from build123d import *

# Parameters (mm, degrees)
SKETCH_1_W          = 99.999995276
SKETCH_1_H          = 99.999995276
SKETCH_1_R          = 7
EXTRUDE_2_DEPTH     = 4
FILLET_2_R          = 7
EXTRUDE_3_DEPTH     = 116
FILLET_3_R          = 3
FILLET_4_R          = 1
CUT_EXTRUDE_1_DEPTH = 116
RIB_1_REACH         = 141.284
SKETCH_6_WALL_W     = 331.945026876
SKETCH_6_WALL_H     = 3


with BuildPart() as part:
    # 草图1 → 凸台-拉伸2 (new body)
    with BuildSketch(Plane(origin=(0, 0, 0), x_dir=(1, 0, 0), z_dir=(0, 1, 0))):
        Rectangle(SKETCH_1_W, SKETCH_1_H)
        with Locations(Location((-35, 35, 0), (0, 0, 270))):
            Circle(SKETCH_1_R, mode=Mode.SUBTRACT)
        with Locations(Location((35, 35, 0), (0, 0, 270))):
            Circle(SKETCH_1_R, mode=Mode.SUBTRACT)
        with Locations(Location((35, -35, 0), (0, 0, 270))):
            Circle(SKETCH_1_R, mode=Mode.SUBTRACT)
        with Locations(Location((-35, -35, 0), (0, 0, 270))):
            Circle(SKETCH_1_R, mode=Mode.SUBTRACT)
    extrude(amount=EXTRUDE_2_DEPTH)

    # 圆角2
    fillet_2_edges = [part.edges().sort_by_distance(p)[0] for p in [
        (-49.999997638, 2, -49.999997638),
        (49.999997638, 2, -49.999997638),
        (49.999997638, 2, 49.999997638),
        (-49.999997638, 2, 49.999997638),
    ]]
    fillet(fillet_2_edges, radius=FILLET_2_R)

    # 草图3 → 凸台-拉伸3 (add)
    with BuildSketch(Plane(origin=(0, 4, 0), x_dir=(1, 0, 0), z_dir=(0, 1, 0))):
        Polygon((-21, -24), (-21, -21), (21, -21), (21, 21), (-21, 21), (-21, 24), (24, 24), (24, -24), align=None)
    extrude(amount=EXTRUDE_3_DEPTH)

    # 圆角3
    fillet_3_edges = [part.edges().sort_by_distance(p)[0] for p in [
        (-21, 120, 22.5),
        (-21, 120, -22.5),
    ]]
    fillet(fillet_3_edges, radius=FILLET_3_R)

    # 圆角4
    fillet_4_edges = [part.edges().sort_by_distance(p)[0] for p in [
        (24, 62, 24),
        (24, 62, -24),
        (21, 62, -21),
        (21, 62, 21),
    ]]
    fillet(fillet_4_edges, radius=FILLET_4_R)

    # 草图4 → 切除-拉伸1 (cut)
    with BuildSketch(Plane(origin=(0, 0, -24), x_dir=(-1, 0, 0), z_dir=(0, 0, -1))):
        with BuildLine():
            Line((4.5, 93.761812865), (4.5, 71.261812865))
            ThreePointArc((4.5, 71.261812865), (0, 66.761812865), (-4.5, 71.261812865))
            Line((-4.5, 71.261812865), (-4.5, 93.761812865))
            ThreePointArc((-4.5, 93.761812865), (0, 98.261812865), (4.5, 93.761812865))
        make_face()
        with BuildLine():
            Line((4.5, 42.026719912), (4.5, 19.526719912))
            ThreePointArc((4.5, 19.526719912), (0, 15.026719912), (-4.5, 19.526719912))
            Line((-4.5, 19.526719912), (-4.5, 42.026719912))
            ThreePointArc((-4.5, 42.026719912), (0, 46.526719912), (4.5, 42.026719912))
        make_face()
    extrude(amount=-CUT_EXTRUDE_1_DEPTH, mode=Mode.SUBTRACT)

    # 草图6 wall → 筋1 (add, up to next)
    with BuildSketch(Plane(origin=(35.249998819, 27.094227832, 0), x_dir=(0.437936853183, -0.89900573559, 0), z_dir=(0.89900573559, 0.437936853183, 0)), mode=Mode.PRIVATE) as rib_1_sk1:
        Rectangle(SKETCH_6_WALL_W, SKETCH_6_WALL_H)
    rib_1_tool1 = extrude(rib_1_sk1.sketch, amount=-RIB_1_REACH, mode=Mode.PRIVATE) - part.part
    add(rib_1_tool1.solids().sort_by_distance((35.249998819, 27.094227832, 0))[0])


solid = part.part
Input: part model. Units: mm. Frame: model coordinates. A direction names the side the tool comes from. Coordinates: 2 decimals unless noted, no trailing zeros. Loops run counter-clockwise (first coordinate to the right, second up) from the corner with the lowest first, then second, coordinate; pieces in that order, holes last. Notation, with made-up numbers: (54, 12.5) -> (74, 12.5) arc R20 ccw to (74, 31.5) -> close; hole circle Ø6 at (30, 10). An arc over 180 degrees is marked (long way). Write item = value, one per line. Start each with the question number.
Item 1: Cut plane A-A, the plane x = 0. Return loops of the section in (y, z), plus the area to 3 significant figures.
Item 2: First-contact query: P1, Ø2.5, axis at y = 25, z = 22.5, coming from the +X side; P2, Ø0.9, axis at y = 26.5, z = -22, coming from the -X side; P3, Ø12, axis at x = 9.5, y = 36.5, coming from the +Z side; P4, Ø12.5, axis at x = 35, z = 35, coming from the +Y side. Flat tips, straight axial feed; report the tip coordinate or a pass-through.
Item 3: Cut plane B-B, the plane z = -35. Return loops of the section in (x, y).
Item 4: Reachability of faces 1 (the face through (-0.099, 15.028, -22.521)), 2 (the face through (24, 61, 0)), 3 (the face through (-21, 60, -22)) from +Z, -Z, +X, -X, +Y, -Y: full face, straight path, thin tool, end or side. Return the list, or none.
Item 5: Mould query, pull axis Y, two halves, no side actions, for faces 4 (the face through (-20.14, 119.1, -22.52)), 5 (the face through (-21, 60, 23)), 6 (the face through (0.099, 46.526, -22.521)). Classes: pulls with the +Y half, pulls with the -Y half, needs draft (parallel to the pull), parting line crosses it, or undercut.
Item 6: Material intervals for line 1 (X direction, y = 2, z = 35); line 2 (Z direction, x = -13.5, y = 41.5); line 3 (X direction, y = 68.5, z = -17), sorted ascending.
Item 7: Cut plane D-D, the plane y = 26. Return loops of the section in (x, z).
Item 8: Cut plane C-C, the plane x = -35. Return loops of the section in (y, z).
Ans:
q1.outline = (0, -50) -> (4, -50) -> (4, -24) -> (15.03, -24) -> (15.03, -21) -> (4, -21) -> (4, 21) -> (15.03, 21) -> (15.03, 24) -> (4, 24) -> (4, 50) -> (0, 50) -> close; (46.53, -24) -> (66.76, -24) -> (66.76, -21) -> (46.53, -21) -> close; (46.53, 21) -> (66.76, 21) -> (66.76, 24) -> (46.53, 24) -> close; (98.26, -24) -> (120, -24) -> (120, -21) -> (98.26, -21) -> close; (98.26, 21) -> (120, 21) -> (120, 24) -> (98.26, 24) -> close
q1.area = 718 mm²
q2.P1 = 24
q2.P2 = -21
q2.P3 = 24
q2.P4 = through
q3.outline = (-50, 0) -> (-42, 0) -> (-42, 4) -> (-50, 4) -> close; (-28, 0) -> (28, 0) -> (28, 4) -> (-28, 4) -> close; (42, 0) -> (50, 0) -> (50, 4) -> (42, 4) -> close
q4.face_1 = +Z, -Z
q4.face_2 = +X, +Y
q4.face_3 = +Z, -Z, -X, +Y
q5.face_4 = pulls with the +Y half
q5.face_5 = needs draft
q5.face_6 = undercut
q6.line_1 = -50 to -42, -28 to 28, 42 to 50
q6.line_2 = -24 to -21, 21 to 24
q6.line_3 = 21 to 24
q7.outline = (-21, -24) -> (-4.5, -24) -> (-4.5, -21) -> (-21, -21) -> close; (-21, 21) -> (-4.5, 21) -> (-4.5, 24) -> (-21, 24) -> close; (4.5, -24) -> (23, -24) arc R1 ccw to (24, -23) -> (24, -1.5) -> (35.78, -1.5) -> (35.78, 1.5) -> (24, 1.5) -> (24, 23) arc R1 ccw to (23, 24) -> (4.5, 24) -> (4.5, 21) -> (20, 21) arc R1 cw to (21, 20) -> (21, -20) arc R1 cw to (20, -21) -> (4.5, -21) -> close
q8.outline = (0, -50) -> (4, -50) -> (4, -42) -> (0, -42) -> close; (0, -28) -> (4, -28) -> (4, 28) -> (0, 28) -> close; (0, 42) -> (4, 42) -> (4, 50) -> (0, 50) -> close
